```python
from build123d import *

# Parameters (mm, degrees)
SKETCH1_W               = 170
SKETCH1_H               = 130
BOSS_EXTRUDE1_DEPTH     = 6
BOSS_EXTRUDE2_DEPTH     = 60
SKETCH3_R               = 9
CUT_EXTRUDE1_DEPTH      = 2.6
FILLET1_R               = 20
MIRROR3_COPY_1_SKETCH_R = 9
MIRROR3_COPY_1_DEPTH    = 2.6
SKETCH5_W               = 105.147186258
SKETCH5_H               = 10
CUT_EXTRUDE2_DEPTH      = 60
CUT_EXTRUDE3_DEPTH      = 6
FILLET2_R               = 5
CUT_EXTRUDE6_DEPTH      = 6


with BuildPart() as part:
    # Sketch1 → Boss-Extrude1 (new body)
    with BuildSketch(Plane(origin=(0, 0, 0), x_dir=(1, 0, 0), z_dir=(0, 1, 0))):
        Rectangle(SKETCH1_W, SKETCH1_H)
    extrude(amount=BOSS_EXTRUDE1_DEPTH)

    # Sketch2 → Boss-Extrude2 (add)
    with BuildSketch(Plane(origin=(0, 6, 0), x_dir=(1, 0, 0), z_dir=(0, 1, 0))):
        Polygon((-75, -32.573593129), (-75, 0), (-85, 0), (-85, -65), (85, -65), (85, 0), (75, 0), (75, -32.573593129), (52.573593129, -55), (45, -55), (-45, -55), (-52.573593129, -55), align=None)
    boss_extrude2 = extrude(amount=BOSS_EXTRUDE2_DEPTH)

    # Mirror1: Boss-Extrude2 across plane
    add(boss_extrude2.mirror(Plane.XY))

    # Sketch3 → Cut-Extrude1 (cut)
    with BuildSketch(Plane(origin=(0, 66, 0), x_dir=(1, 0, 0), z_dir=(0, 1, 0))):
        with Locations(Location((-73, 53, 0), (0, 0, 270))):
            Circle(SKETCH3_R)
    cut_extrude1 = extrude(amount=-CUT_EXTRUDE1_DEPTH, mode=Mode.SUBTRACT)

    # Fillet1
    fillet1_edges = [part.edges().sort_by_distance(p)[0] for p in [
        (-75, 36, 32.573593129),
        (75, 36, 32.573593129),
        (-75, 36, -32.573593129),
        (-52.573593129, 36, -55),
        (52.573593129, 36, -55),
        (75, 36, -32.573593129),
    ]]
    fillet(fillet1_edges, radius=FILLET1_R)

    # Mirror2: Cut-Extrude1 across plane
    add(cut_extrude1.mirror(Plane(origin=(0, 0, 0), x_dir=(0, 0, 1), z_dir=(1, 0, 0))), mode=Mode.SUBTRACT)

    # Mirror3: Cut-Extrude1 across plane
    add(cut_extrude1.mirror(Plane.XY), mode=Mode.SUBTRACT)

    # Mirror3 copy 1 sketch → Mirror3 copy 1 (cut)
    with BuildSketch(Plane(origin=(0, 66, 0), x_dir=(-1, 0, 0), z_dir=(0, 1, 0))):
        with Locations(Location((-73, 53, 0), (0, 0, 270))):
            Circle(MIRROR3_COPY_1_SKETCH_R)
    extrude(amount=-MIRROR3_COPY_1_DEPTH, mode=Mode.SUBTRACT)

    # Sketch5 → Cut-Extrude2 (cut)
    with BuildSketch(Plane(origin=(0, 66, 0), x_dir=(1, 0, 0), z_dir=(0, 1, 0))):
        with Locations((0, -60)):
            Rectangle(SKETCH5_W, SKETCH5_H)
    extrude(amount=-CUT_EXTRUDE2_DEPTH, mode=Mode.SUBTRACT)

    # Sketch7 → Cut-Extrude3 (cut)
    with BuildSketch(Plane(origin=(85, 0, 0), x_dir=(0, 0, -1), z_dir=(1, 0, 0))):
        Polygon((-55, 15), (-55, 45), (-50, 45), (-44, 36.838679983), (-44, 29.838679983), (-50, 38), (-50, 15), align=None)
        Polygon((-33.090970614, 22), (-33.090970614, 45), (-28.090970614, 45), (-28.090970614, 15), (-33.090970614, 15), (-39.090970614, 23.161320017), (-39.090970614, 30.161320017), align=None)
        with BuildLine():
            Line((1.909029386, 45), (-2.090970614, 45))
            ThreePointArc((-2.090970614, 45), (0.030349729, 44.121320344), (0.909029386, 42))
            Line((0.909029386, 42), (0.909029386, 18))
            ThreePointArc((0.909029386, 18), (0.030349729, 15.878679656), (-2.090970614, 15))
            Line((-2.090970614, 15), (1.909029386, 15))
            ThreePointArc((1.909029386, 15), (4.030349729, 15.878679656), (4.909029386, 18))
            Line((4.909029386, 18), (4.909029386, 42))
            ThreePointArc((4.909029386, 42), (4.030349729, 44.121320344), (1.909029386, 45))
        make_face()
        with BuildLine():
            Line((-21.090970614, 42), (-21.090970614, 18))
            ThreePointArc((-21.090970614, 18), (-20.212290958, 15.878679656), (-18.090970614, 15))
            Line((-18.090970614, 15), (-14.090970614, 15))
            ThreePointArc((-14.090970614, 15), (-16.212290958, 15.878679656), (-17.090970614, 18))
            Line((-17.090970614, 18), (-17.090970614, 42))
            ThreePointArc((-17.090970614, 42), (-16.212290958, 44.121320344), (-14.090970614, 45))
            Line((-14.090970614, 45), (-18.090970614, 45))
            ThreePointArc((-18.090970614, 45), (-20.212290958, 44.121320344), (-21.090970614, 42))
        make_face()
        Polygon((11.909029386, 45), (11.909029386, 15), (22.909029386, 15), (35.516776739, 45), (30.516776739, 45), (19.909029386, 19), (16.909029386, 19), (16.909029386, 45), align=None)
        Polygon((31.347758846, 15), (43.9555062, 45), (55, 45), (54.340720725, 15), (49.339513512, 15), (49.867454564, 39.023554456), (46.867454564, 39.023554456), (36.771357727, 15), align=None)
        with BuildLine():
            Line((-4.624822618, 15), (-11.090970614, 15))
            ThreePointArc((-11.090970614, 15), (-13.212290958, 15.878679656), (-14.090970614, 18))
            Line((-14.090970614, 18), (-14.090970614, 42))
            ThreePointArc((-14.090970614, 42), (-13.212290958, 44.121320344), (-11.090970614, 45))
            Line((-11.090970614, 45), (-4.624822618, 45))
            ThreePointArc((-4.624822618, 45), (-2.503502275, 44.121320344), (-1.624822618, 42))
            Line((-1.624822618, 42), (-1.624822618, 18))
            ThreePointArc((-1.624822618, 18), (-2.503502275, 15.878679656), (-4.624822618, 15))
        make_face()
    extrude(amount=-CUT_EXTRUDE3_DEPTH, mode=Mode.SUBTRACT)

    # Fillet2
    fillet2_edges = [part.edges().sort_by_distance(p)[0] for p in [
        (85, 33, 65),
        (-85, 33, 65),
    ]]
    fillet(fillet2_edges, radius=FILLET2_R)

    # Sketch12 → Cut-Extrude6 (cut)
    with BuildSketch(Plane.ZY.offset(85)):
        Polygon((-39, 47), (-35, 47), (-30.482690446, 31.238340543), (-23.885743409, 47), (-19.599215517, 47), (-32.155533692, 17), (-36.491760677, 17), (-33, 25.342638252), align=None)
        Polygon((-14.599215517, 47), (-27.155533692, 17), (-23.155533692, 17), (-12.210225245, 43.791772221), (-8.210225245, 43.791772221), (-8.210225245, 17), (-4.210225245, 17), (-4.210225245, 47), align=None)
        Polygon((-37, 25.342638252), (-43, 47), (-47, 47), (-41, 25.342638252), (-44.491760677, 17), (-40.491760677, 17), align=None)
        Polygon((0.789774755, 47), (0.789774755, 17), (4.789774755, 17), (4.789774755, 30), (13.888047314, 30), (13.888047314, 34), (4.789774755, 34), (4.789774755, 43), (13.888047314, 43), (13.888047314, 47), align=None)
        Polygon((20.27200974, 47), (24.27200974, 47), (31.13600487, 36.933214608), (38, 47), (42, 47), (42, 43), (34.499696428, 32), (42, 21), (42, 17), (38, 17), (31.13600487, 27.066785392), (24.27200974, 17), (20.27200974, 17), (12.245273414, 17), (12.245273414, 21), (20.27200974, 21), (27.772313311, 32), (20.27200974, 43), align=None)
    extrude(amount=-CUT_EXTRUDE6_DEPTH, mode=Mode.SUBTRACT)


solid = part.part
```
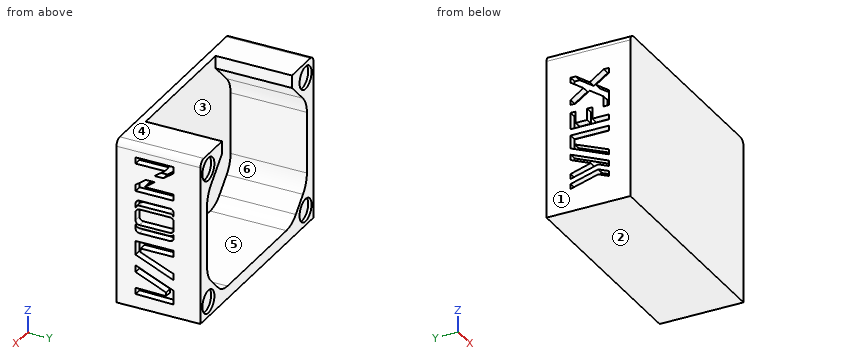
Design review of the part built by this model. Coordinates are the model's own, in mm. Face numbers are marked on the shaded views. A direction names the side the tool comes from. Coordinates: 2 decimals unless noted, no trailing zeros. Write each loop counter-clockwise with the first axis right and the second up, starting at its lowest first coordinate (ties: lowest second). Pieces come first, ordered by that corner, then holes. Notation, with made-up numbers: M 7.5,72.25 L 37.5,72.25 A17 ccw 37.5,104.25 Z; hole C -2,66 d3. An arc over 180 degrees is marked long. Answer as a JSON object with one key per item and string values.
Item 1: Machinability: for the marked faces 4, 5 and 6, which of the approach directions +Z, -Z, +X, -X, +Y, -Y give a long, thin tool a straight path to every point of the face, cutting with its end or side? Answer none if there is none.
Outcome:
{"face 4": "+Z, +X, -X, +Y, -Y", "face 5": "+Z, +Y", "face 6": "+Y"}
Item 2: Add section C-C, the plane x = -3.5. Give the boundary of the cut face in (y, z), and give its area (3 significant figures).
Outcome:
{"outline": "M 0,-65 L 66,-65 L 66,-55 L 6,-55 L 6,65 L 0,65 Z", "area": "1,380 mm²"}
Item 3: Add section D-D, the plane x = 73. Give the boundary of the cut face in (y, z).
Outcome:
{"outline": "M 0,-65 L 66,-65 L 66,-62 L 63.4,-62 L 63.4,-44 L 66,-44 L 66,-33.01 L 6,-33.01 L 6,33.01 L 66,33.01 L 66,44 L 63.4,44 L 63.4,62 L 66,62 L 66,65 L 0,65 Z"}
Item 4: Insertion check: pin 1 Ø4 at (x, y) = (11.5, 42.5) entering from +Z; pin 2 Ø3 at (y, z) = (47.5, 62.5) entering from +X. Each pin has a flat end and moves straight along its axis. Give the tip position at first contact, or say it passes through.
Outcome:
{"pin 1": "z = -55", "pin 2": "x = 84.9"}
Item 5: Draft analysis for pull direction X (two halves, no side actions). For the marked faces 1, 2 and 3, state which applies: pulls with the +X half, pulls with the -X half, needs draft (parallel to the pull), parting line crosses it, or undercut.
Outcome:
{"face 1": "pulls with the -X half", "face 2": "needs draft", "face 3": "undercut"}
Item 6: Add section B-B, the plane z = 53. Give the boundary of the cut face in (x, y).
Outcome:
{"outline": "M -85,0 L 85,0 L 85,15 L 79,15 L 79,45 L 85,45 L 85,66 L 82,66 L 82,63.4 L 64,63.4 L 64,66 L 54.57,66 L 54.57,6 L -54.57,6 L -54.57,66 L -64,66 L -64,63.4 L -82,63.4 L -82,66 L -85,66 Z"}
Item 7: Add section A-A, the plane y = 10.5. Give the boundary of the cut face in (x, z).
Outcome:
{"outline": "M -85,-65 L 85,-65 L 85,60 A5 ccw 80,65 L 52.57,65 L 52.57,55 L 69.14,38.43 A20 cw 75,24.29 L 75,-24.29 A20 cw 69.14,-38.43 L 58.43,-49.14 A20 cw 44.29,-55 L -44.29,-55 A20 cw -58.43,-49.14 L -69.14,-38.43 A20 cw -75,-24.29 L -75,24.29 A20 cw -69.14,38.43 L -52.57,55 L -52.57,65 L -80,65 A5 ccw -85,60 Z"}
Item 8: Wall thickness on probe 1 along X at (y, z) = (53, -4.5); probe 2 along X at (y, z) = (65.05, -53); probe 3 along Z at (x, y) = (73, 65.35): over which ranges is each line inside the solid? List them lowest first.
Outcome:
{"probe 1": "-85 to -75, 75 to 85", "probe 2": "-85 to -82, -64 to -53.01, 53.01 to 64, 82 to 85", "probe 3": "-65 to -62, -44 to -33.01, 33.01 to 44, 62 to 65"}
